from build123d import *

# Parameters (mm, degrees)
SKETCH1_W           = 292
SKETCH1_H           = 150
BOSS_EXTRUDE1_DEPTH = 8
SKETCH2_R           = 6
CUT_EXTRUDE1_DEPTH  = 165.331981063
SKETCH3_R           = 7.5
CUT_EXTRUDE2_DEPTH  = 165.331981063


with BuildPart() as part:
    # Sketch1 → Boss-Extrude1 (new body)
    with BuildSketch(Plane(origin=(0, 0, 0), x_dir=(0, 1, 0), z_dir=(0, 0, 1))):
        Rectangle(SKETCH1_W, SKETCH1_H)
    extrude(amount=BOSS_EXTRUDE1_DEPTH)

    # Sketch2 → Cut-Extrude1 (cut, through all)
    with BuildSketch(Plane.XY.offset(8)):
        with Locations((-55, 55)):
            Circle(SKETCH2_R)
        with Locations((55, 55)):
            Circle(SKETCH2_R)
        with Locations((-55, -55)):
            Circle(SKETCH2_R)
        with Locations((55, -55)):
            Circle(SKETCH2_R)
    extrude(amount=-CUT_EXTRUDE1_DEPTH, mode=Mode.SUBTRACT)

    # Sketch3 → Cut-Extrude2 (cut, through all)
    with BuildSketch(Plane(origin=(0, 0, 0), x_dir=(0, 1, 0), z_dir=(0, 0, 1))):
        with Locations(Location((0, 0, 0), (0, 0, 270))):
            Circle(SKETCH3_R)
    extrude(amount=CUT_EXTRUDE2_DEPTH, mode=Mode.SUBTRACT)


solid = part.part
For this review, take the finished solid that the model builds, in its own axes (mm). Coordinates: 2 decimals unless noted, no trailing zeros. Order: outer loops, then holes, each group sorted by start corner. A loop starts at its lowest first (then second) coordinate and runs counter-clockwise, first axis right, second up. Notation, with made-up numbers: (33, 87) -> (57, 87) arc R6 cw to (57, 93) -> close; hole circle Ø5 at (-15, 29.25). An arc over 180 degrees is marked (long way). Return JSON: item names as keys, results as strings.
1. For line 1 (Y direction, x = 55, z = 2.25); line 2 (X direction, y = 0, z = 2.75); line 3 (Y direction, x = -56, z = 4.5), list the stretches that pass through material, from the lowest coordinate up. Write a range as from..to.
Answer block:
{"line 1": "-146..-61, -49..49, 61..146", "line 2": "-75..-7.5, 7.5..75", "line 3": "-146..-60.92, -49.08..49.08, 60.92..146"}
2. We need section C-C on x = 55. Write out the cut boundary in (y, z), and give its area (3 significant figures).
Answer block:
{"outline": "(-146, 0) -> (-61, 0) -> (-61, 8) -> (-146, 8) -> close; (-49, 0) -> (49, 0) -> (49, 8) -> (-49, 8) -> close; (61, 0) -> (146, 0) -> (146, 8) -> (61, 8) -> close", "area": "2,140 mm²"}
3. The part is to be moulded in two halves that separate along X. For faces 1 (the cylindrical face through (-7.493, 0.33, 3.944)), 2 (the flat face through (75, -2, 4)), 3 (the flat face through (1, -146, 4)), say which applies: +X half, -X half, draft (parallel to the pull), parting line (faces both ways), or undercut.
Answer block:
{"face 1": "undercut", "face 2": "+X half", "face 3": "draft"}
4. We need section A-A on y = -55. Write out the cut boundary in (x, z).
Answer block:
{"outline": "(-75, 0) -> (-61, 0) -> (-61, 8) -> (-75, 8) -> close; (-49, 0) -> (49, 0) -> (49, 8) -> (-49, 8) -> close; (61, 0) -> (75, 0) -> (75, 8) -> (61, 8) -> close"}
5. We need section B-B on x = 0. Write out the cut boundary in (y, z).
Answer block:
{"outline": "(-146, 0) -> (-7.5, 0) -> (-7.5, 8) -> (-146, 8) -> close; (7.5, 0) -> (146, 0) -> (146, 8) -> (7.5, 8) -> close"}
